Part model, mm, in its own coordinate system. Coordinates: 2 decimals unless noted, no trailing zeros. Order: outer loops, then holes, each group sorted by start corner. A loop starts at its lowest first (then second) coordinate and runs counter-clockwise, first axis right, second up. Notation, with made-up numbers: (61.5, 65.25) - (107.5, 65.25) arc R22 ccw to (107.5, 103.25) - close; hole circle Ø8 at (61, 35). An arc over 180 degrees is marked (long way). Use a Markdown table: item, result. Add a question column.
1) Saw through at B-B on y = 6.5. List the corners of the cut face in (x, z), then the cut area to 3 significant figures.
2) Drop flat-ended pins along their axis: P1, Ø1, axis at x = 4, z = 14, coming from the -Y side; P2, Ø5, axis at y = -13, z = 13, coming from the +X side; P3, Ø6, axis at y = -15, z = 36.5, coming from the +X side. Give the stop position or say it passes through.
3) Saw through at C-C on x = -5. List the corners of the cut face in (y, z), then the cut area to 3 significant figures.
4) Saw through at A-A on z = 24.5. List the corners of the cut face in (x, y).
5) Two-plate mould, pull along X, no slides. Class faces 1 (the face through (0, -1, 100)), 2 (the face through (-79.274, 6.277, 49.3)), 3 (the face through (71.766, -34.291, 49.3)): +X half, -X half, draft (parallel to the pull), parting line (faces both ways), or undercut.
6) Wall check: L1, parallel to Y at x = 50, z = 18; L2, parallel to Y at x = -49, z = 44.5. Give the ranges that are in metal, low to high. Write a range as [from, to].
```python
from build123d import *

# Parameters (mm, degrees)
BOSS_EXTRUDE1_DEPTH = 100


with BuildPart() as part:
    # Sketch1 → Boss-Extrude1 (new body)
    with BuildSketch(Plane(origin=(0, 0, 0), x_dir=(-1, 0, 0), z_dir=(0, 0, 1))):
        with BuildLine():
            Line((67.973290008, -37.656184374), (68.004301332, -37.570981461))
            ThreePointArc((68.004301332, -37.570981461), (68.797575177, -36.575628395), (70.030727156, -36.260434305))
            Line((70.030727156, -36.260434305), (78.47997961, -9.462829137))
            Line((78.47997961, -9.462829137), (80.091350343, -2.999974125))
            ThreePointArc((80.091350343, -2.999974125), (79.982164163, -1.81678638), (79.159491845, -0.959426994))
            ThreePointArc((79.159491845, -0.959426994), (77.685261787, -0.04212625), (76.391925323, 1.116353663))
            Line((76.391925323, 1.116353663), (-65.599171142, 39.162753293))
            ThreePointArc((-65.599171142, 39.162753293), (-67.298473332, 38.806148491), (-69.033844385, 38.748857773))
            ThreePointArc((-69.033844385, 38.748857773), (-70.174979205, 38.417698923), (-70.861131083, 37.447621369))
            Line((-70.861131083, 37.447621369), (-72.6970706, 31.044939381))
            Line((-72.6970706, 31.044939381), (-78.778605915, 3.612906317))
            ThreePointArc((-78.778605915, 3.612906317), (-77.86826202, 2.723364239), (-77.678943251, 1.464726275))
            Line((-77.678943251, 1.464726275), (-77.694688113, 1.375432727))
            ThreePointArc((-77.694688113, 1.375432727), (-77.453437445, 0.021779086), (-76.395283749, -0.8562248))
            ThreePointArc((-76.395283749, -0.8562248), (-76.393715257, -0.986290661), (-76.391925323, -1.116353663))
            Line((-76.391925323, -1.116353663), (65.599171142, -39.162753293))
            ThreePointArc((65.599171142, -39.162753293), (65.665752771, -39.051010396), (65.732144056, -38.939154303))
            ThreePointArc((65.732144056, -38.939154303), (67.08753398, -38.707857481), (67.973290008, -37.656184374))
        make_face()
    extrude(amount=BOSS_EXTRUDE1_DEPTH)


solid = part.part
```
Results are:
| question | item | result |
|---|---|---|
| 1 | outline | (-79.22, 0) - (56.3, 0) - (56.3, 100) - (-79.22, 100) - close |
| 1 | area | 13,600 mm2 |
| 2 | P1 | y = -22.79 |
| 2 | P2 | x = 77.25 |
| 2 | P3 | x = 76.92 |
| 3 | outline | (-20.25, 0) - (22.93, 0) - (22.93, 100) - (-20.25, 100) - close |
| 3 | area | 4,320 mm2 |
| 4 | outline | (-80.09, 3) arc R1.8 ccw to (-79.16, 0.96) arc R10 cw to (-76.39, -1.12) - (65.6, -39.16) arc R10 cw to (69.03, -38.75) arc R1.8 ccw to (70.86, -37.45) - (72.7, -31.04) - (78.78, -3.61) arc R2 cw to (77.68, -1.46) - (77.69, -1.38) arc R2 ccw to (76.4, 0.86) arc R76.4 ccw to (76.39, 1.12) - (-65.6, 39.16) arc R76.4 ccw to (-65.73, 38.94) arc R2 ccw to (-67.97, 37.66) - (-68, 37.57) arc R2 cw to (-70.03, 36.26) - (-78.48, 9.46) - close |
| 5 | face 1 | draft |
| 5 | face 2 | -X half |
| 5 | face 3 | +X half |
| 6 | L1 | [-34.98, 8.19] |
| 6 | L2 | [-8.46, 34.72] |
